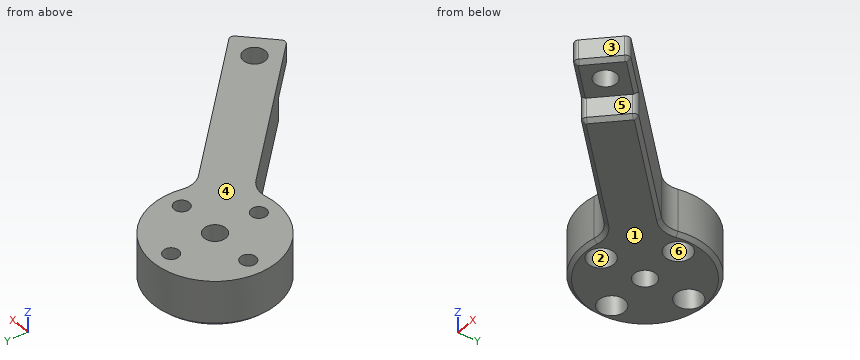
from build123d import *

# Parameters (mm, degrees)
SKETCH002_R     = 2.35
SKETCH002_R_2   = 1.65
PAD001_DEPTH    = 10
POCKET001_DEPTH = 5
SKETCH004_R     = 2.8
POCKET002_DEPTH = 5
FILLET004_R     = 5
FILLET005_R     = 1
CHAMFER009_SIZE = 0.8


with BuildPart() as part:
    # Sketch002 → Pad001 (new body)
    with BuildSketch(Plane.XY):
        with BuildLine():
            Line((0, 7.071068), (-22.952731, 30.023799))
            ThreePointArc((-22.952731, 30.023799), (-44.901281, 44.901281), (-30.023799, 22.952731))
            Line((-7.071068, 0), (-30.023799, 22.952731))
            Line((-7.071068, 0), (0, -7.071068))
            Line((0, -7.071068), (7.071068, 0))
            Line((7.071068, 0), (0, 7.071068))
        make_face()
        Circle(SKETCH002_R, mode=Mode.SUBTRACT)
        with Locations((-44.855339, 35.355339)):
            Circle(SKETCH002_R_2, mode=Mode.SUBTRACT)
        with Locations((-25.855339, 35.355339)):
            Circle(SKETCH002_R_2, mode=Mode.SUBTRACT)
        with Locations((-35.355339, 25.855339)):
            Circle(SKETCH002_R_2, mode=Mode.SUBTRACT)
        with Locations((-35.355339, 44.855339)):
            Circle(SKETCH002_R_2, mode=Mode.SUBTRACT)
        with Locations((-35.355339, 35.355339)):
            Circle(SKETCH002_R, mode=Mode.SUBTRACT)
    extrude(amount=PAD001_DEPTH)

    # Sketch003 (on Face13 of Pad001) → Pocket001 (cut)
    with BuildSketch(Plane(origin=(0, 0, 0), x_dir=(1, 0, 0), z_dir=(0, 0, -1))):
        Polygon((0, 7.071068), (-7.071068, 0), (0, -7.071068), (7.071068, 0), align=None)
    extrude(amount=-POCKET001_DEPTH, mode=Mode.SUBTRACT)

    # Sketch004 (on Face13 of Pad001) → Pocket002 (cut)
    with BuildSketch(Plane(origin=(0, 0, 0), x_dir=(1, 0, 0), z_dir=(0, 0, -1))):
        with Locations((-44.855339, -35.355339)):
            Circle(SKETCH004_R)
        with Locations((-35.355339, -25.855339)):
            Circle(SKETCH004_R)
        with Locations((-25.855339, -35.355339)):
            Circle(SKETCH004_R)
        with Locations((-35.355339, -44.855339)):
            Circle(SKETCH004_R)
    extrude(amount=-POCKET002_DEPTH, mode=Mode.SUBTRACT)

    # Fillet004
    fillet004_edges = [part.edges().sort_by_distance(p)[0] for p in [
        (-22.952731, 30.023799, 5),
        (-30.023799, 22.952731, 5),
    ]]
    fillet(fillet004_edges, radius=FILLET004_R)

    # Fillet005
    fillet005_edges = [part.edges().sort_by_distance(p)[0] for p in [
        (7.071068, 0, 7.5),
        (0, -7.071068, 7.5),
        (0, 7.071068, 2.5),
        (-7.071068, 0, 2.5),
    ]]
    fillet(fillet005_edges, radius=FILLET005_R)

    # Chamfer009
    chamfer009_edges = [part.edges().sort_by_distance(p)[0] for p in [
        (-3.535534, 3.535534, 0),
        (3.535534, -3.535534, 5),
    ]]
    chamfer(chamfer009_edges, length=CHAMFER009_SIZE)


with BuildPart() as part_1:
    # Body001 placement: moved
    add(part.part.moved(Location((-62, 61.9, 0.6))))


solid = part_1.part
For this review, take the finished solid that the model builds, in its own axes (mm). Face numbers are marked on the shaded views. A direction names the side the tool comes from. Round coordinates to 2 decimals unless told otherwise and drop trailing zeros. Order: outer loops, then holes, each group sorted by start corner. A loop starts at its lowest first (then second) coordinate and runs counter-clockwise, first axis right, second up. Notation, with made-up numbers: (88, 15) -> (122, 15) arc R34 cw to (122, 47) -> close; hole circle Ø6 at (34, 76). An arc over 180 degrees is marked (long way). Put each result on its own line as item: value.
Q1. Machinability: for the marked faces 4, 5 and 6, which of the approach directions +Z, -Z, +X, -X, +Y, -Y give a long, thin tool a straight path to every point of the face, cutting with its end or side? Answer none if there is none.
Check result:
face 4: +Z, +X, -X, +Y, -Y
face 5: -Z, +X, -Y
face 6: -Z
Q2. Add section A-A on z = 8.75. Write out the cut boundary in (x, y), plus the area to 3 significant figures.
Check result:
outline: (-94.48, 84.06) arc R5 cw to (-89.89, 82.71) -> (-62.71, 55.54) arc R1 ccw to (-61.29, 55.54) -> (-55.64, 61.19) arc R1 ccw to (-55.64, 62.61) -> (-82.81, 89.79) arc R5 cw to (-84.16, 94.38) arc R13.5 ccw (long way) to start; hole circle Ø3.3 at (-106.86, 97.26); hole circle Ø4.7 at (-97.36, 97.26); hole circle Ø3.3 at (-97.36, 87.76); hole circle Ø3.3 at (-97.36, 106.76); hole circle Ø3.3 at (-87.86, 97.26); hole circle Ø4.7 at (-62, 61.9)
area: 924 mm2
Q3. Add section C-C on y = 66.5. Write out the cut boundary in (x, z).
Check result:
outline: (-73.67, 1.4) -> (-72.54, 0.6) -> (-65.6, 0.6) -> (-64.47, 1.4) -> (-64.47, 5.6) -> (-60.66, 5.6) -> (-59.53, 6.4) -> (-59.53, 10.6) -> (-73.67, 10.6) -> close
Q4. Insertion check: pin 1 Ø4.5 at (x, y) = (-87.86, 97.26) entering from -Z; pin 2 Ø1 at (y, z) = (63.5, 9.5) entering from +X; pin 3 Ø2 at (y, z) = (79.5, 5.5) entering from -X. Each pin has a flat end and moves straight along its axis. Give the tip position at first contact, or say it passes through.
Check result:
pin 1: z = 5.6
pin 2: x = -56.03
pin 3: x = -87.67
Q5. Add section D-D on y = 81. Write out the cut boundary in (x, z).
Check result:
outline: (-88.17, 1.4) -> (-87.04, 0.6) -> (-75.16, 0.6) -> (-74.03, 1.4) -> (-74.03, 10.6) -> (-88.17, 10.6) -> close
Q6. For probe 1 along X at (y, z) = (97, 8.25); probe 2 along X at (y, z) = (88, 3.75); probe 3 along X at (y, z) = (104.5, 2.25), list the stretches that pass through material, from the lowest coordinate up. Write a range as [from, to].
Check result:
probe 1: [-110.85, -108.49], [-105.23, -99.69], [-95.02, -89.49], [-86.23, -83.86]
probe 2: [-107.18, -100.14], [-94.57, -81.03]
probe 3: [-108.75, -99.01], [-95.7, -85.96]
Q7. Mouldability with a two-part tool opening along Y and no side actions: class the marked faces 1, 2 and 3 as pulls with the +Y half, pulls with the -Y half, needs draft (parallel to the pull), parting line crosses it, or undercut.
Check result:
face 1: needs draft
face 2: undercut
face 3: pulls with the -Y half
Q8. Add section B-B on x = -78. Write out the cut boundary in (y, z), plus the area to 3 significant figures.
Check result:
outline: (70.83, 1.4) -> (71.96, 0.6) -> (83.84, 0.6) -> (84.97, 1.4) -> (84.97, 10.6) -> (70.83, 10.6) -> close
area: 141 mm2
